Input: dimensioned drawing with shaded views. Units: mm. Origin: part minimum x, y, z. Coordinates: 2 decimals unless noted, no trailing zeros. Write each loop counter-clockwise with the first axis right and the second up, starting at its lowest first coordinate (ties: lowest second). Pieces come first, ordered by that corner, then holes. Notation, with made-up numbers: M 2.5,21 L 49.5,21 A15 ccw 49.5,34 Z; hole C 13,-26 d5. An arc over 180 degrees is marked long. Use one line per item in the form item = value.
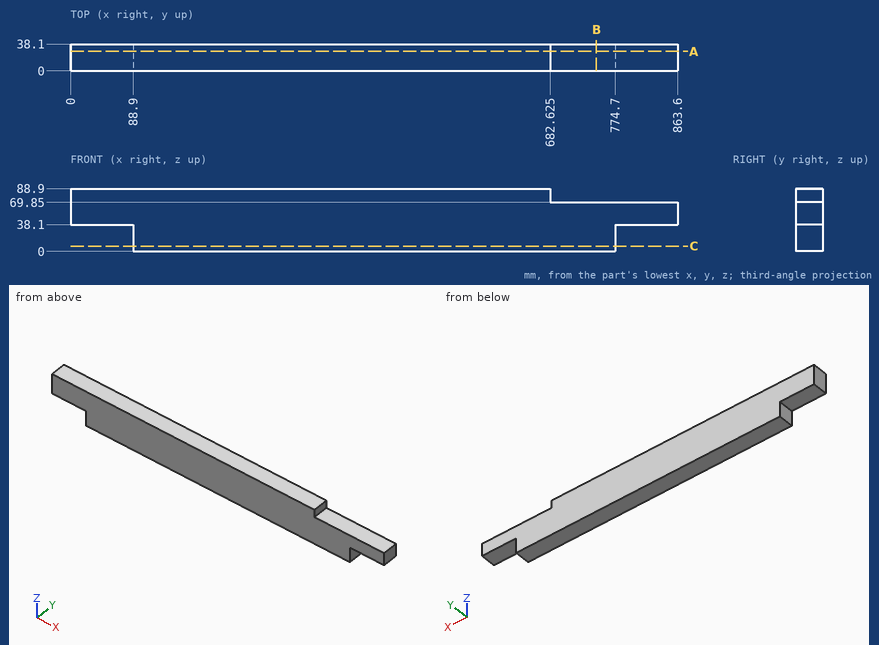
(1) Section query A-A on y = 27.5. Return the cut outline in (x, z) (3 decimals), plus the area to 3 significant figures.
Computed:
outline = M 0,38.1 L 88.9,38.1 L 88.9,0 L 774.7,0 L 774.7,38.1 L 863.6,38.1 L 863.6,69.85 L 682.625,69.85 L 682.625,88.9 L 0,88.9 Z
area = 66,600 mm^2
(2) Section query B-B on x = 748. Return the cut outline in (y, z), plus the area to 3 significant figures.
Computed:
outline = M 0,0 L 38.1,0 L 38.1,69.85 L 0,69.85 Z
area = 2,660 mm^2
(3) Line query: probe 1 along X at (y, z) = (13.5, 27.5); probe 2 along Z at (x, y) = (689.5, 31.5); probe 3 along X at (y, z) = (18, 72.5) (3 decimals). Output: solid intervals per line, ascending.
Computed:
probe_1 = 88.9 to 774.7
probe_2 = 0 to 69.85
probe_3 = 0 to 682.625
(4) First-contact query: pin 1 Ø10 at (y, z) = (17.5, 79.5) entering from +X (3 decimals); pin 2 Ø8 at (y, z) = (23.5, 19) entering from -X; pin 3 Ø11.5 at (x, y) = (763, 17.5) entering from +Z. Flat tips, straight axial feed; report the tip coordinate or a pass-through.
Computed:
pin_1 = 682.625
pin_2 = 88.9
pin_3 = 69.85
(5) Section query C-C on z = 7.5. Return the cut outline in (x, y), plus the area to 3 significant figures.
Computed:
outline = M 88.9,0 L 774.7,0 L 774.7,38.1 L 88.9,38.1 Z
area = 26,100 mm^2
